The listing builds one solid part. Answer for the finished solid, in the listing's coordinates (mm). Face numbers are marked on the shaded views. A direction names the side the tool comes from. Coordinates: 2 decimals unless noted, no trailing zeros. Loops run counter-clockwise (first coordinate to the right, second up) from the corner with the lowest first, then second, coordinate; pieces in that order, holes last. Notation, with made-up numbers: M -28.75,49 L 18.25,49 A14 ccw 18.25,61 Z; hole C 65,65 d2. An arc over 180 degrees is marked long. Answer as a JSON object with one key per item and string values. Group by question number.
1. A cutting plane is placed at C-C on y = 0. Give the vertices of the cut face in (x, z).
2. For the marked faces 4 and 5, determine the directions among +Z, -Z, +X, -X, +Y, -Y from which every point of the face is accessible in a straight line to the end or side of a thin tool.
3. Determine the mould class of the marked faces 1, 2 and 3 for opening direction X: released by +X, released by -X, zero draft, split by the parting line, or undercut.
4. Given pin 1 (3 mm diameter, centred on x = 1, y = -10, fed in from +Z), flat-ended and moving along its own axis, determine where the tip first touches the part or whether it passes through.
5. A cutting plane is placed at A-A on y = -8.75. Give the vertices of the cut face in (x, z).
6. Straight lines are drawn through the part: L1, parallel to X at y = 0, z = 0.55; L2, parallel to X at y = -3.25, z = 1.9; L3, parallel to Y at x = 0, z = 1.6. For each, find the intervals that lie inside material, in ascending order.
7. A cutting plane is placed at B-B on z = 1.6. Give the vertices of the cut face in (x, y), and give its area (3 significant figures).
8. A cutting plane is placed at D-D on x = 0. Give the vertices of the cut face in (y, z), and give its area (3 significant figures).
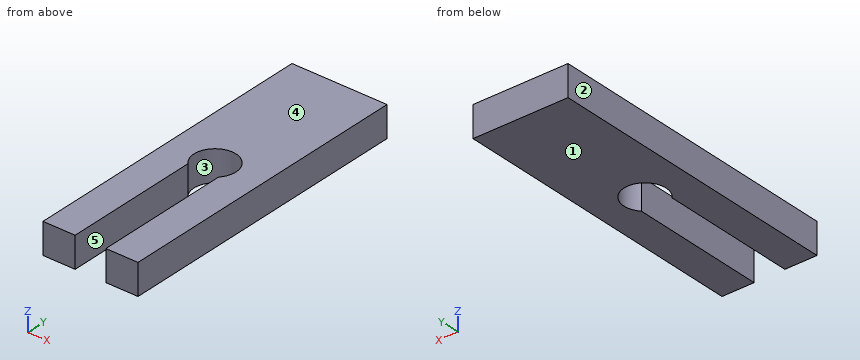
from build123d import *

# Parameters (mm, degrees)
SKETCH032_W     = 8
SKETCH032_H     = 25.4
PAD005_DEPTH    = 2.6
POCKET031_DEPTH = 2.601
SKETCH035_R     = 1.7685
POCKET032_DEPTH = 2.901


with BuildPart() as part:
    # Sketch032 → Pad005 (new body)
    with BuildSketch(Plane.XY):
        Rectangle(SKETCH032_W, SKETCH032_H)
    extrude(amount=PAD005_DEPTH)

    # Sketch033 (on Face5 of Pad005) → Pocket031 (cut, through all)
    with BuildSketch(Plane(origin=(0, 0, 0), x_dir=(1, 0, 0), z_dir=(0, 0, -1))):
        with BuildLine():
            ThreePointArc((-1.294, 0), (0, -1.294), (1.294, 0))
            Line((1.294, 0), (1.294, 12.7))
            Line((1.294, 12.7), (-1.294, 12.7))
            Line((-1.294, 12.7), (-1.294, 0))
        make_face()
    extrude(amount=-POCKET031_DEPTH, mode=Mode.SUBTRACT)

    # Sketch035 → Pocket032 (cut, through all)
    with BuildSketch(Plane.XY.offset(2.9)):
        Circle(SKETCH035_R)
    extrude(amount=-POCKET032_DEPTH, mode=Mode.SUBTRACT)


solid = part.part
From the geometry:
{
 "1": {"outline": "M -4,0 L -1.77,0 L -1.77,2.6 L -4,2.6 Z; M 1.77,0 L 4,0 L 4,2.6 L 1.77,2.6 Z"},
 "2": {"face 4": "+Z, +X, -X, +Y, -Y", "face 5": "+Z, -Z, -Y"},
 "3": {"face 1": "zero draft", "face 2": "released by -X", "face 3": "undercut"},
 "4": {"pin 1": "stops at z = 2.6"},
 "5": {"outline": "M -4,0 L -1.29,0 L -1.29,2.6 L -4,2.6 Z; M 1.29,0 L 4,0 L 4,2.6 L 1.29,2.6 Z"},
 "6": {"L1": "x = -4 to -1.77, 1.77 to 4", "L2": "x = -4 to -1.29, 1.29 to 4", "L3": "y = 1.77 to 12.7"},
 "7": {"outline": "M -4,-12.7 L -1.29,-12.7 L -1.29,-1.21 A1.77 cw long 1.29,-1.21 L 1.29,-12.7 L 4,-12.7 L 4,12.7 L -4,12.7 Z", "area": "165 mm²"},
 "8": {"outline": "M 1.77,0 L 12.7,0 L 12.7,2.6 L 1.77,2.6 Z", "area": "28.4 mm²"}
}
